Input: part model. Units: mm. Frame: model coordinates. A direction names the side the tool comes from. Round coordinates to 2 decimals unless told otherwise and drop trailing zeros. Order: outer loops, then holes, each group sorted by start corner. A loop starts at its lowest first (then second) coordinate and runs counter-clockwise, first axis right, second up.
Item 1: Reachability of faces 4 (the flat face through (160, 98, 8)), 5 (the flat face through (-3, 6, 0)), 6 (the flat face through (207, 10, 8)), 7 (the flat face through (-105, -55, 7)), 8 (the flat face through (-208, 50, 8)) from +Z, -Z, +X, -X, +Y, -Y: full face, straight path, thin tool, end or side. Return the list, or none.
Item 2: Cut plane B-B on x = -65.5. Output: boundary loops of the cut face in (y, z), then the cut area to 3 significant figures.
Item 3: First-contact query: pin 1 (6 mm diameter, centred on y = 83.5, z = 12, fed in from -X); pin 2 (4.5 mm diameter, centred on x = 24.5, z = 10, fed in from +Y); pin 3 (2 mm diameter, centred on x = 162.5, z = 6.5, fed in from +Y). Flat tips, straight axial feed; report the tip coordinate or a pass-through.
Item 4: Mould query, pull axis X, two halves, no side actions, for faces 1 (the flat face through (215, 77, 8)), 2 (the flat face through (-207, 10, 8)), 3 (the flat face through (-120, 97, 8)). Classes: released by +X, released by -X, zero draft, split by the parting line, or undercut.
Item 5: Cut plane A-A on x = -110.5. Output: boundary loops of the cut face in (y, z).
Item 6: Line query: L1, parallel to Y at x = 190, z = 6; L2, parallel to X at y = 47.5, z = 6; L3, parallel to X at y = -21, z = 8.75. Output: solid intervals per line, ascending.
```python
from build123d import *

# Parameters (mm, degrees)
SALIENTE_EXTRUIR1_DEPTH = 15
CROQUIS2_W              = 430
CROQUIS2_H              = 15
SALIENTE_EXTRUIR2_DEPTH = 15
CROQUIS3_W              = 40
CROQUIS3_H              = 19.65418827
CORTAR_EXTRUIR2_DEPTH   = 15
CORTAR_EXTRUIR3_DEPTH   = 15
CORTAR_EXTRUIR4_DEPTH   = 15


with BuildPart() as part:
    # Croquis1 → Saliente-Extruir1 (new body)
    with BuildSketch(Plane.XY):
        Polygon((95, -45), (140, -90), (215, -90), (215, -20), (215, 90), (-215, 90), (-215, -20), (-215, -90), (-140, -90), (-95, -45), (-70, -20), (70, -20), align=None)
    extrude(amount=SALIENTE_EXTRUIR1_DEPTH)

    # Croquis2 → Saliente-Extruir2 (add)
    with BuildSketch(Plane(origin=(0, 90, 0), x_dir=(1, 0, 0), z_dir=(0, 1, 0))):
        with Locations((0, -7.5)):
            Rectangle(CROQUIS2_W, CROQUIS2_H)
    extrude(amount=SALIENTE_EXTRUIR2_DEPTH)

    # Croquis3 → Cortar-Extruir2 (cut)
    with BuildSketch(Plane.XY.offset(15)):
        with Locations((-140, 114.827094135)):
            Rectangle(CROQUIS3_W, CROQUIS3_H)
        with BuildLine():
            Line((-120, 90), (-120, 105))
            Line((-120, 105), (-160, 105))
            Line((-160, 105), (-160, 90))
            ThreePointArc((-160, 90), (-156.75, 86.75), (-153.5, 90))
            Line((-153.5, 90), (-126.5, 90))
            ThreePointArc((-126.5, 90), (-123.25, 86.75), (-120, 90))
        make_face()
        with BuildLine():
            Line((-40, 90), (-40, 105))
            Line((-40, 105), (-80, 105))
            Line((-80, 105), (-80, 90))
            ThreePointArc((-80, 90), (-76.75, 86.75), (-73.5, 90))
            Line((-73.5, 90), (-46.5, 90))
            ThreePointArc((-46.5, 90), (-43.25, 86.75), (-40, 90))
        make_face()
        with Locations((-60, 114.827094135)):
            Rectangle(CROQUIS3_W, CROQUIS3_H)
        with BuildLine():
            Line((40, 105), (0, 105))
            Line((0, 105), (0, 90))
            ThreePointArc((0, 90), (3.25, 86.75), (6.5, 90))
            Line((6.5, 90), (33.5, 90))
            ThreePointArc((33.5, 90), (36.75, 86.75), (40, 90))
            Line((40, 90), (40, 105))
        make_face()
        with Locations((20, 114.827094135)):
            Rectangle(CROQUIS3_W, CROQUIS3_H)
        with BuildLine():
            Line((200, 105), (160, 105))
            Line((160, 105), (160, 90))
            ThreePointArc((160, 90), (163.25, 86.75), (166.5, 90))
            Line((166.5, 90), (193.5, 90))
            ThreePointArc((193.5, 90), (196.75, 86.75), (200, 90))
            Line((200, 90), (200, 105))
        make_face()
        with Locations((180, 114.827094135)):
            Rectangle(CROQUIS3_W, CROQUIS3_H)
        with Locations((100, 114.827094135)):
            Rectangle(CROQUIS3_W, CROQUIS3_H)
        with BuildLine():
            Line((120, 105), (80, 105))
            Line((80, 105), (80, 90))
            ThreePointArc((80, 90), (83.25, 86.75), (86.5, 90))
            Line((86.5, 90), (113.6, 90))
            ThreePointArc((113.6, 90), (116.8, 86.8), (120, 90))
            Line((120, 90), (120, 105))
        make_face()
    extrude(amount=-CORTAR_EXTRUIR2_DEPTH, mode=Mode.SUBTRACT)

    # Croquis4 → Cortar-Extruir3 (cut)
    with BuildSketch(Plane.XY.offset(15)):
        with BuildLine():
            Line((-200, 10), (-215, 10))
            Line((-215, 10), (-215, -30))
            Line((-215, -30), (-200, -30))
            ThreePointArc((-200, -30), (-196.75, -26.75), (-200, -23.5))
            Line((-200, -23.5), (-200, 3.5))
            ThreePointArc((-200, 3.5), (-196.75, 6.75), (-200, 10))
        make_face()
        with BuildLine():
            Line((-215, 90), (-215, 50))
            Line((-215, 50), (-200, 50))
            ThreePointArc((-200, 50), (-196.75, 53.25), (-200, 56.5))
            Line((-200, 56.5), (-200, 83.5))
            ThreePointArc((-200, 83.5), (-196.75, 86.75), (-200, 90))
            Line((-200, 90), (-215, 90))
        make_face()
    extrude(amount=-CORTAR_EXTRUIR3_DEPTH, mode=Mode.SUBTRACT)

    # Croquis5 → Cortar-Extruir4 (cut)
    with BuildSketch(Plane.XY.offset(15)):
        with BuildLine():
            Line((215, 10), (215, 50))
            Line((215, 50), (200, 50))
            ThreePointArc((200, 50), (196.75, 46.75), (200, 43.5))
            Line((200, 43.5), (200, 16.5))
            ThreePointArc((200, 16.5), (196.75, 13.25), (200, 10))
            Line((200, 10), (215, 10))
        make_face()
        with BuildLine():
            Line((215, -70), (215, -30))
            Line((215, -30), (200, -30))
            ThreePointArc((200, -30), (196.75, -33.25), (200, -36.5))
            Line((200, -36.5), (200, -63.5))
            ThreePointArc((200, -63.5), (196.75, -66.75), (200, -70))
            Line((200, -70), (215, -70))
        make_face()
    extrude(amount=-CORTAR_EXTRUIR4_DEPTH, mode=Mode.SUBTRACT)


solid = part.part
```
From the geometry:
1. face 4: +Z, -Z, +Y
1. face 5: -Z, +X, -X, +Y, -Y
1. face 6: +Z, -Z, +X
1. face 7: +Z, -Z, -Y
1. face 8: +Z, -Z, -X
2. outline: (-20, 0) - (90, 0) - (90, 15) - (-20, 15) - close
2. area: 1,650 mm2
3. pin 1: stops at x = -200
3. pin 2: stops at y = 90
3. pin 3: stops at y = 87.26
4. face 1: released by +X
4. face 2: zero draft
4. face 3: undercut
5. outline: (-60.5, 0) - (105, 0) - (105, 15) - (-60.5, 15) - close
6. L1: y = -90 to 90
6. L2: x = -215 to 196.84
6. L3: x = -200 to -71, 71 to 215
